Study the drawing (mm; zero at the part's minimum x, y, z) and answer. A direction names the side the tool comes from. Give positions to 0.01 mm unless a question says otherwise; leave off trailing zeros. Order: outer loops, then holes, each group sorted by start corner. A loop starts at its lowest first (then second) coordinate and runs counter-clockwise, first axis right, second up.
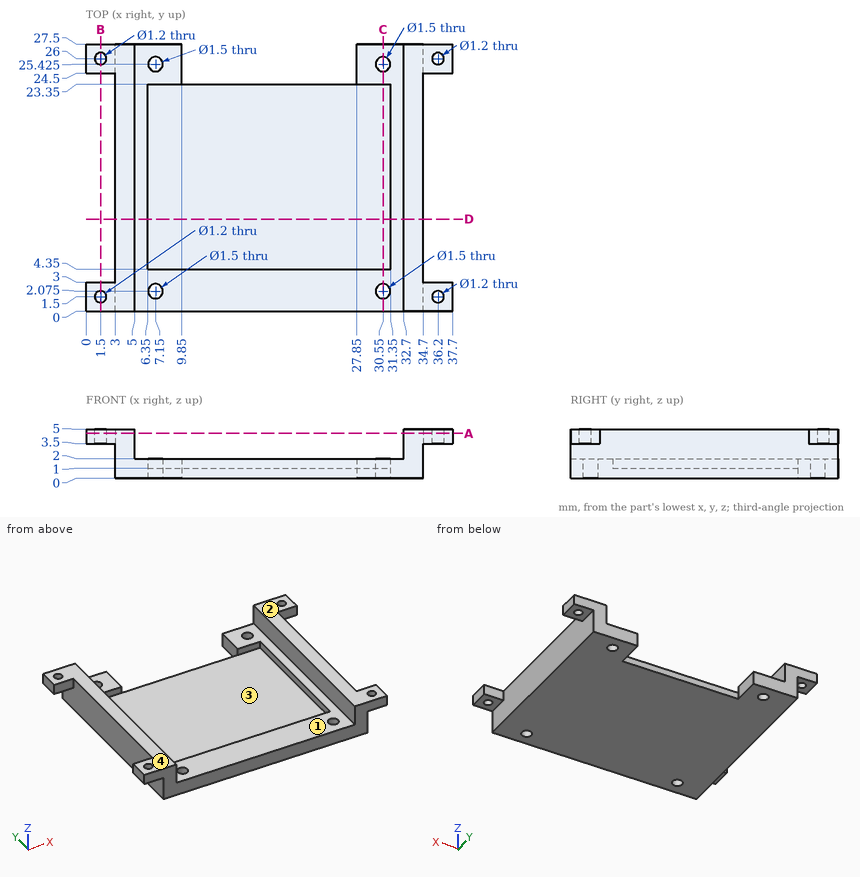
1) Find section B-B (x = 1.5). Write down the section's boundary in (y, z).
Geometry says:
outline: (0, 3.5) - (0.9, 3.5) - (0.9, 5) - (0, 5) - close; (2.1, 3.5) - (3, 3.5) - (3, 5) - (2.1, 5) - close; (24.5, 3.5) - (25.4, 3.5) - (25.4, 5) - (24.5, 5) - close; (26.6, 3.5) - (27.5, 3.5) - (27.5, 5) - (26.6, 5) - close
2) Find section C-C (x = 30.55). Write down the section's boundary in (y, z) (3 decimals).
Geometry says:
outline: (0, 0) - (1.325, 0) - (1.325, 2) - (0, 2) - close; (2.825, 0) - (24.675, 0) - (24.675, 2) - (23.35, 2) - (23.35, 1) - (4.35, 1) - (4.35, 2) - (2.825, 2) - close; (26.175, 0) - (27.5, 0) - (27.5, 2) - (26.175, 2) - close
3) A tool of negligible diameter and unlimited length cuts with its end or side. For the marked faces 3 and 4, from which of +Z, -Z, +X, -X, +Y, -Y can it reach the whole face along a straight path? Write none if from no direction.
Geometry says:
face 3: +Z
face 4: +Z, +X, -X, +Y, -Y
4) For a pull along X with two mould halves and no side action, classify the marked faces 1 and 2 as +X half, -X half, draft (parallel to the pull), parting line (faces both ways), or undercut.
Geometry says:
face 1: undercut
face 2: draft
5) Find section D-D (y = 9.5). Write down the section's boundary in (x, z).
Geometry says:
outline: (3, 0) - (34.7, 0) - (34.7, 5) - (32.7, 5) - (32.7, 2) - (31.35, 2) - (31.35, 1) - (6.35, 1) - (6.35, 2) - (5, 2) - (5, 5) - (3, 5) - close
6) Straight lines are drawn through the part: probe 1 along Y at (x, z) = (1.5, 4.45); probe 2 along Y at (x, z) = (30.55, 1.4) (3 decimals); probe 3 along X at (y, z) = (26, 4.6). For each, find the intervals that lie inside material, in ascending order.
Geometry says:
probe 1: y = 0 to 0.9, 2.1 to 3, 24.5 to 25.4, 26.6 to 27.5
probe 2: y = 0 to 1.325, 2.825 to 4.35, 23.35 to 24.675, 26.175 to 27.5
probe 3: x = 0 to 0.9, 2.1 to 5, 32.7 to 35.6, 36.8 to 37.7
7) Find section A-A (z = 4.6). Write down the section's boundary in (x, y), then the cut area to 3 significant figures.
Geometry says:
outline: (0, 0) - (5, 0) - (5, 27.5) - (0, 27.5) - (0, 24.5) - (3, 24.5) - (3, 3) - (0, 3) - close; (32.7, 0) - (37.7, 0) - (37.7, 3) - (34.7, 3) - (34.7, 24.5) - (37.7, 24.5) - (37.7, 27.5) - (32.7, 27.5) - close; hole circle Ø1.2 at (1.5, 1.5); hole circle Ø1.2 at (1.5, 26); hole circle Ø1.2 at (36.2, 1.5); hole circle Ø1.2 at (36.2, 26)
area: 141 mm2
8) Given P1, Ø1, axis at y = 19, z = 3, coming from the -X side; P2, Ø0.9, axis at x = 1, y = 26, coming from the -Z side; P3, Ø0.7, axis at x = 36.2, y = 26, coming from the +Z side; P4, Ø1.5, axis at y = 14, z = 1.5, coming from the +X side, each flat-ended and moving along its own axis, determine where each tip first touches the part or whether it passes through.
Geometry says:
P1: stops at x = 3
P2: stops at z = 3.5
P3: passes through
P4: stops at x = 34.7
